Design review of the part built by this model. Coordinates are the model's own, in mm. A direction names the side the tool comes from. Coordinates: 2 decimals unless noted, no trailing zeros. Order: outer loops, then holes, each group sorted by start corner. A loop starts at its lowest first (then second) coordinate and runs counter-clockwise, first axis right, second up. Notation, with made-up numbers: M -9,-20 L 24,-20 A14 cw 24,-13 Z; hole C 56.5,-1 d10. An arc over 180 degrees is marked long. Answer as a JSON object with one key per item and string values.
Autodesk Inventor part; units mm, degrees
ref_plane "YZ Plane" through (0, 0, 0) normal (1, 0, 0) x (0, 1, 0)
ref_plane "XZ Plane" through (0, 0, 0) normal (0, 1, 0) x (-1, 0, 0)
ref_plane "XY Plane" through (0, 0, 0) normal (0, 0, 1) x (1, 0, 0)
sketch "Sketch1" plane through (0, 0, 0) normal (1, 0, 0) x (0, 1, 0)
  line L0 (14, 25) -> (-14, 25)
  line L1 (-14, 25) -> (-14, -25)
  line L2 (-14, -25) -> (14, -25)
  line L3 (14, -25) -> (14, 25)
  point P0 (0, 0)
  dimension "d0" = 50
  dimension "d1" = 25
  dimension "d2" = 28
  dimension "d3" = 14
extrude "Extrusion1" add sketch "Sketch1" against normal blind 5
sketch "Sketch2" plane through (0, 0, 0) normal (1, 0, 0) x (0, 0, -1)
  circle A0 centre (-12.1, 10.5) radius 0.55
  circle A1 centre (-14.95, 10.5) radius 1
  circle A2 centre (4.25, 10.5) radius 0.55
  circle A3 centre (7.1, 10.5) radius 1
  line L0 (25, -14) -> (25, 14)
  line L1 (-25, 14) -> (-25, -14)
  line L2 (-14.95, 10.5) -> (7.1, 10.5) construction
  line L3 (-25, -14) -> (25, -14)
  line L4 (25, 14) -> (-25, 14)
  line L5 (-8.2421, 4) -> (2.4524, 4) construction
  circle A4 centre (-12.1, -2.5) radius 0.55
  circle A5 centre (-14.95, -2.5) radius 1
  circle A6 centre (4.25, -2.5) radius 0.55
  circle A7 centre (7.1, -2.5) radius 1
  line L6 (-14.95, -2.5) -> (7.1, -2.5) construction
  point P0 (0, 0)
  dimension "d6" = 2
  dimension "d7" = 2
  dimension "d8" = 1.1
  dimension "d9" = 1.1
  dimension "d11" = 2.85
  dimension "d13" = 2.85
  dimension "d14" = 10.05
  dimension "d19" = 16.35
  dimension "d20" = 3.5
  dimension "d28" = 10
extrude "Extrusion2" cut sketch "Sketch2" against normal up to surface (5 mm away) contours A0 | A1 | A2 | A3 | A4 | A5 | A6 | A7
fillet "Fillet1" radius 0.5 8 edges at (0, 0, 25) (0, 14, 0) (0, 0, -25) (0, -14, 0) (-2.5, 14, 25) (-2.5, -14, 25) (-2.5, 14, -25) (-2.5, -14, -25)
sketch "Sketch3" plane through (0, 0, 0) normal (1, 0, 0) x (0, 0, -1)
  line L0 (-22.5, 12.5) -> (22.6, 12.5)
  line L1 (22.6, 12.5) -> (22.6, 0.5)
  line L2 (22.6, 0.5) -> (-22.5, 0.5)
  line L3 (-22.5, 0.5) -> (-22.5, 12.5)
  circle A0 centre (-14.95, 10.5) radius 1
  line L4 (0, 0) -> (3.2775, 0) construction
  line L5 (-22.5, -12.5) -> (22.6, -12.5)
  line L6 (22.6, -12.5) -> (22.6, -0.5)
  line L7 (22.6, -0.5) -> (-22.5, -0.5)
  line L8 (-22.5, -0.5) -> (-22.5, -12.5)
  dimension "d21" = 45.1
  dimension "d22" = 7.55
  dimension "d23" = 10
  dimension "d24" = 2
extrude "Extrusion3" cut sketch "Sketch3" against normal blind 0.1
properties part number "Dual_Backplate"
1) Mouldability with a two-part tool opening along Z and no side actions: class faces 1 (the flat face through (-3, 0, 25)), 2 (the flat face through (-0.1, -6, 0)), 3 (the flat face through (-3, 0, -25)) as released by +Z, released by -Z, zero draft, split by the parting line, or undercut.
Taken from the geometry:
{"face 1": "released by +Z", "face 2": "undercut", "face 3": "released by -Z"}
2) Insertion check: pin 1 Ø3.5 at (y, z) = (7.5, 1.5) entering from +X; pin 2 Ø2.5 at (y, z) = (-2.5, -7.1) entering from -X; pin 3 Ø1.8 at (y, z) = (10.5, 14.95) entering from -X. Each pin has a flat end and moves straight along its axis. Give the tip position at first contact, or say it passes through.
Taken from the geometry:
{"pin 1": "stops at x = -0.1", "pin 2": "stops at x = -5", "pin 3": "passes through"}
3) Add section A-A (z = 12.1). State the section outline as (x, y) points, and give its area (3 significant figures).
Taken from the geometry:
{"outline": "M -5,-14 L -0.5,-14 A0.5 ccw 0,-13.5 L 0,-12.5 L -0.1,-12.5 L -0.1,-3.05 L -5,-3.05 Z; M -5,-1.95 L -0.1,-1.95 L -0.1,-0.5 L 0,-0.5 L 0,0.5 L -0.1,0.5 L -0.1,9.95 L -5,9.95 Z; M -5,11.05 L -0.1,11.05 L -0.1,12.5 L 0,12.5 L 0,13.5 A0.5 ccw -0.5,14 L -5,14 Z", "area": "127 mm2"}
4) Add section C-C (z = 19). State the section outline as (x, y) points.
Taken from the geometry:
{"outline": "M -5,-14 L -0.5,-14 A0.5 ccw 0,-13.5 L 0,-12.5 L -0.1,-12.5 L -0.1,-0.5 L 0,-0.5 L 0,0.5 L -0.1,0.5 L -0.1,12.5 L 0,12.5 L 0,13.5 A0.5 ccw -0.5,14 L -5,14 Z"}
5) Tool access review of faces 4 (the cylindrical face through (-2.516, -2.335, 11.575)), 5 (the flat face through (-0.1, 7, 0)): name each direction out of +Z, -Z, +X, -X, +Y, -Y from which nothing blocks a thin tool from reaching the whole face with its end or side.
Taken from the geometry:
{"face 4": "+X, -X", "face 5": "+X"}
6) Add section B-B (y = 10.5). State the section outline as (x, z) points, and give its area (3 significant figures).
Taken from the geometry:
{"outline": "M -5,-25 L -0.5,-25 A0.5 ccw 0,-24.5 L 0,-22.6 L -0.1,-22.6 L -0.1,-8.1 L -5,-8.1 Z; M -5,-6.1 L -0.1,-6.1 L -0.1,-4.8 L -5,-4.8 Z; M -5,-3.7 L -0.1,-3.7 L -0.1,11.55 L -5,11.55 Z; M -5,12.65 L -0.1,12.65 L -0.1,13.95 L -5,13.95 Z; M -5,15.95 L -0.1,15.95 L -0.1,22.5 L 0,22.5 L 0,24.5 A0.5 ccw -0.5,25 L -5,25 Z", "area": "215 mm2"}
7) To check wall thickness, follow L1, parallel to Y at x = -3.1, z = -4.25; L2, parallel to Y at x = -1.8, z = -7.1; L3, parallel to X at y = 2.75, z = -9. State the ranges of each line that lie inside material, in increasing order.
Taken from the geometry:
{"L1": "y = -14 to -3.05, -1.95 to 9.95, 11.05 to 14", "L2": "y = -14 to -3.5, -1.5 to 9.5, 11.5 to 14", "L3": "x = -5 to -0.1"}
8) Add section D-D (y = -9.75). State the section outline as (x, z) points, and give its area (3 significant figures).
Taken from the geometry:
{"outline": "M -5,-25 L -0.5,-25 A0.5 ccw 0,-24.5 L 0,-22.6 L -0.1,-22.6 L -0.1,22.5 L 0,22.5 L 0,24.5 A0.5 ccw -0.5,25 L -5,25 Z", "area": "245 mm2"}
